Study the drawing (mm; zero at the part's minimum x, y, z) and answer. Round coordinates to 2 decimals unless told otherwise and drop trailing zeros. Write each loop counter-clockwise with the first axis right and the second up, starting at its lowest first coordinate (ties: lowest second). Pieces come first, ordered by that corner, then holes. Notation, with made-up numbers: (44.5, -16.75) - (89.5, -16.75) arc R17 ccw to (89.5, -9.75) - close; hole circle Ø1 at (-38.75, -39). An arc over 180 degrees is marked (long way). Return JSON: item names as keys, results as strings. Group by question number.
(1) Section A-A, the plane z = 224.5 is taken. Write down the section's boundary in (x, y) (3 decimals), then the cut area to 3 significant figures.
(2) Section C-C, the plane y = 1.9 is taken. Give the number of separate pieces and of enclosed holes in the cut face, then the cut area to 3 significant figures.
(3) Find the intervals of material crossed by line 1 along X through (y, z) = (2.05, 203.2); line 2 along Z through (x, y) = (48, 1.15); line 3 along X through (y, z) = (2.1, 6.35), in increasing order. Write a range as [from, to].
(4) Section B-B, the plane x = 50 is taken. Write down the section's boundary in (y, z) (3 decimals).
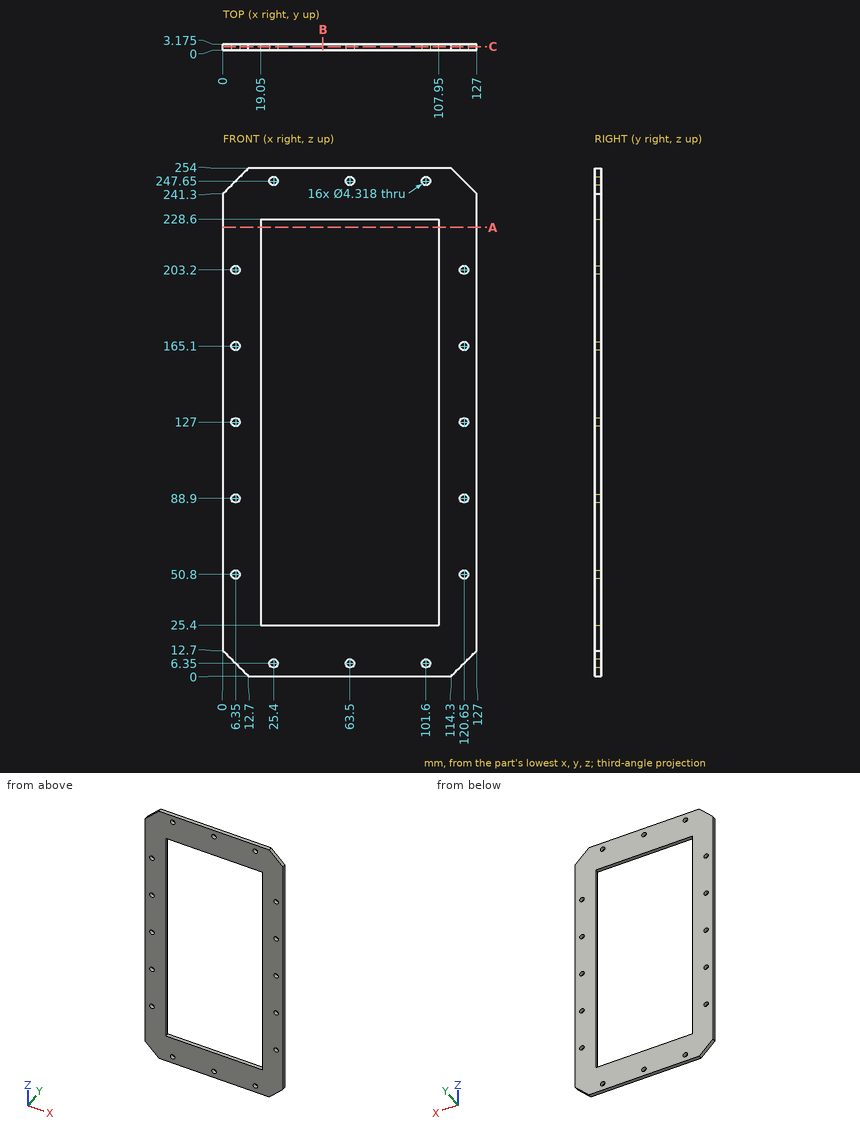
Working result:
{
 "1": {"outline": "(0, 0) - (19.05, 0) - (19.05, 3.175) - (0, 3.175) - close; (107.95, 0) - (127, 0) - (127, 3.175) - (107.95, 3.175) - close", "area": "121 mm^2"},
 "2": {"separate pieces": "1", "enclosed holes": "17", "area": "13,600 mm^2"},
 "3": {"line 1": "x = [0, 4.19], [8.51, 19.05], [107.95, 118.49], [122.81, 127]", "line 2": "z = [0, 25.4], [228.6, 254]", "line 3": "x = [6.35, 23.24], [27.56, 61.34], [65.66, 99.44], [103.76, 120.65]"},
 "4": {"outline": "(0, 0) - (3.175, 0) - (3.175, 25.4) - (0, 25.4) - close; (0, 228.6) - (3.175, 228.6) - (3.175, 254) - (0, 254) - close"}
}
